For this review, use the dimensioned drawing (mm, ordinates from the lowest corner) and the shaded views. Round coordinates to 2 decimals unless told otherwise and drop trailing zeros. Answer in a Markdown table with one row per item. Add a question column.
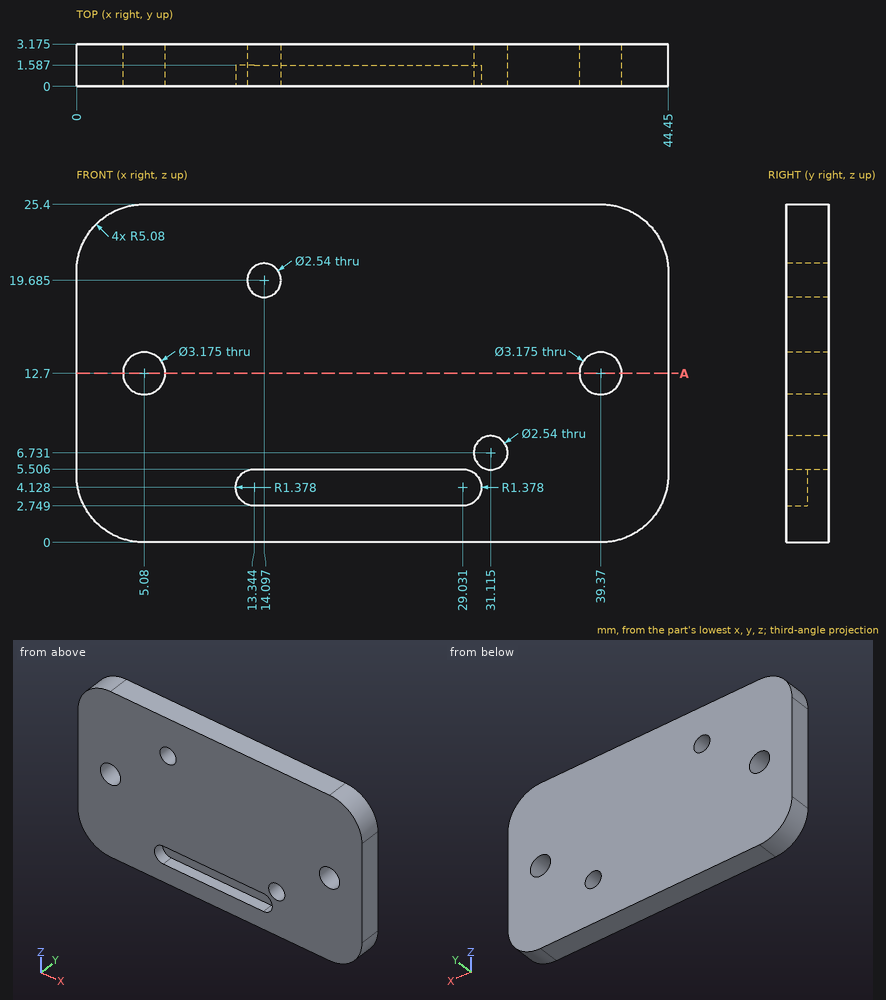
1. We need section A-A (z = 12.7). Count the separate pieces of the cut face and the enclosed holes in it, plus the area to 3 significant figures.
2. Clearance check with a flat-ended pin moving along its axis: pin 1 Ø3.5 at (x, z) = (39.37, 12.7) entering from +Y (1 decimal). State where the tip first meets the part, or that it passes through.
3. For L1, parallel to Z at x = 39.5, y = 0.8; L2, parallel to X at y = 1.75, z = 13; L3, parallel to X at y = 2.55, z = 20.5 (1 decimal), list the stretches that pass through material, from the lowest coordinate up. Write a range as [from, to].
Response:
| question | item | result |
|---|---|---|
| 1 | separate pieces | 3 |
| 1 | enclosed holes | 0 |
| 1 | area | 121 mm2 |
| 2 | pin 1 | y = 3.2 |
| 3 | L1 | [0, 11.12], [14.28, 25.4] |
| 3 | L2 | [0, 3.52], [6.64, 37.81], [40.93, 44.45] |
| 3 | L3 | [0, 13.1], [15.1, 44.4] |
